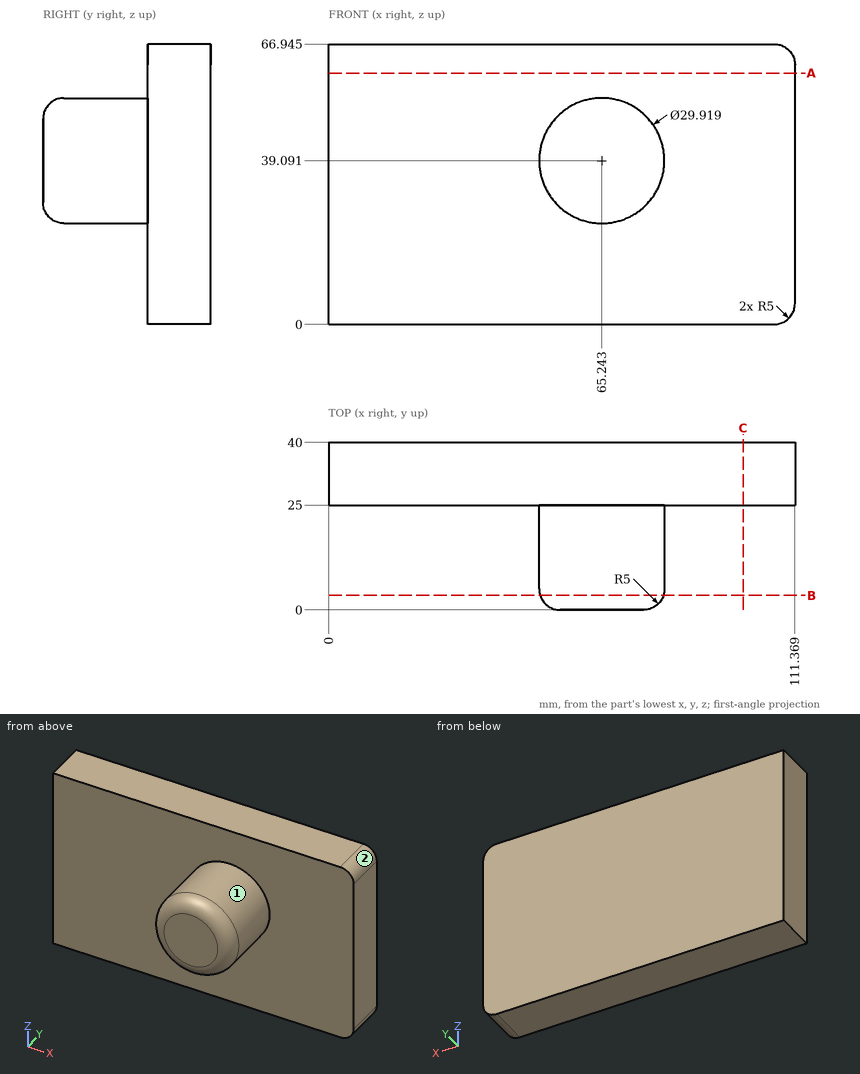
Check sheet for the drawn part. Datum: minimum x, y, z corner. Units: mm. A direction names the side the tool comes from. Coordinates: 2 decimals unless noted, no trailing zeros. Write each loop counter-clockwise with the first axis right and the second up, starting at its lowest first coordinate (ties: lowest second). Pieces come first, ordered by that corner, then holes. Notation, with made-up numbers: M 22,34 L 27,34 A24 cw 27,60 Z; hole C 62.25,82.25 d8. An arc over 180 degrees is marked long. One line per item, written item: value.
Item 1: Section check B-B, the plane y = 3.5. Record the boundary of the cut face in (x, z).
Check sheet entries:
outline: C 65.24,39.09 d29.46
Item 2: Scan lines: line 1 along Y through (x, z) = (41.5, 10.5); line 2 along X through (y, z) = (10.5, 36); line 3 along Z through (x, y) = (53.5, 13) (1 decimal). Record each from-to range of solid material in increasing order.
Check sheet entries:
line 1: y = 25 to 40
line 2: x = 50.61 to 79.88
line 3: z = 29.8 to 48.4
Item 3: Section check C-C, the plane x = 99. Record the boundary of the cut face in (y, z) (1 decimal).
Check sheet entries:
outline: M 25,0 L 40,0 L 40,66.9 L 25,66.9 Z
Item 4: Section check A-A, the plane z = 60. Record the boundary of the cut face in (x, y).
Check sheet entries:
outline: M 0,25 L 111.37,25 L 111.37,40 L 0,40 Z
Item 5: Access from +Z, -Z, +X, -X, +Y, -Y to the whole of each face (thin tool, end or side, straight path). Record for the marked faces 1 and 2.
Check sheet entries:
face 1: -Y
face 2: +Z, +X, +Y, -Y
Item 6: Gauge pin test, flat ends, axial feed: pin 1 Ø10 at (y, z) = (18, 40) entering from -X; pin 2 Ø8 at (y, z) = (13, 27) entering from +X (1 decimal); pin 3 Ø2 at (y, z) = (17.5, 48) entering from +X; pin 4 Ø20 at (x, z) = (59.5, 44.5) entering from -Y. Record the tip position at first contact, or that the pin passes through.
Check sheet entries:
pin 1: stops at x = 50.28
pin 2: stops at x = 77.8
pin 3: stops at x = 77.94
pin 4: stops at y = 0
